Design review of the part built by this model. Coordinates are the model's own, in mm. Give positions to 0.01 mm unless a question says otherwise; leave off trailing zeros. Loops run counter-clockwise (first coordinate to the right, second up) from the corner with the lowest first, then second, coordinate; pieces in that order, holes last.
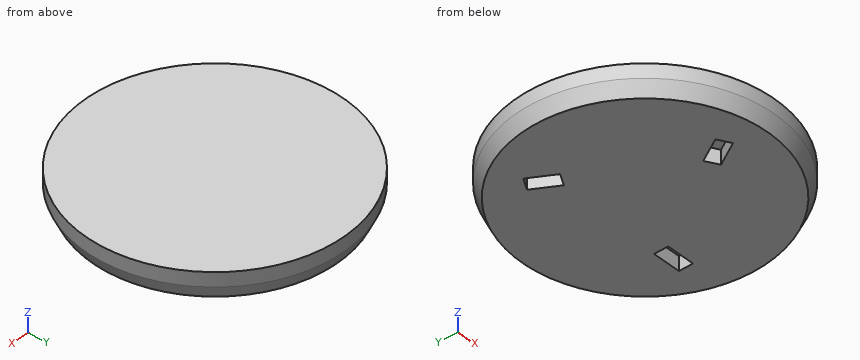
from build123d import *

# Parameters (mm, degrees)
F0_R     = 165
F1_DEPTH = 36
F2_W     = 36
F2_H     = 18
F3_DEPTH = 18
F4_SIZE2 = 8.393538
F4_SIZE  = 18


with BuildPart() as f1:
    # F0 (on Top) → F1 (new body)
    with BuildSketch(Plane.XY):
        Circle(F0_R)
    extrude(amount=F1_DEPTH)

    # F2 (on face) → F3 (cut)
    with BuildSketch(Plane(origin=(0, 0, 0), x_dir=(1, 0, 0), z_dir=(0, 0, -1))):
        Polygon((-9, 120.176915), (-24.588457, 111.176915), (-6.588457, 80), (9, 89), align=None)
        with Locations((90.576261, -43.294229)):
            Rectangle(F2_W, F2_H)
        Polygon((-81.576261, -36.705771), (-99.576261, -67.882686), (-83.987804, -76.882686), (-65.987804, -45.705771), align=None)
    extrude(amount=-F3_DEPTH, mode=Mode.SUBTRACT)

    # F4
    f4_edges = [f1.edges().sort_by_distance(p)[0] for p in [
        (-165, 0, 0),
    ]]
    chamfer(f4_edges, length=F4_SIZE, length2=F4_SIZE2)


solid = f1.part
Q1. Take a section at A-A (z = 12). Give the boundary of the cut face in (x, y).
Results:
outline: circle Ø324.4 at (0, 0); hole (-99.58, 67.88) - (-81.58, 36.71) - (-65.99, 45.71) - (-83.99, 76.88) - close; hole (-24.59, -111.18) - (-9, -120.18) - (9, -89) - (-6.59, -80) - close; hole (72.58, 34.29) - (108.58, 34.29) - (108.58, 52.29) - (72.58, 52.29) - close
Q2. Take a section at B-B (x = 0). Give the boundary of the cut face in (y, z).
Results:
outline: (-165, 18) - (-156.61, 0) - (-104.59, 0) - (-104.59, 18) - (-83.8, 18) - (-83.8, 0) - (156.61, 0) - (165, 18) - (165, 36) - (-165, 36) - close
Q3. Wall thickness on line 1 (Y direction, x = 76.5, z = 5); line 2 (Y direction, x = -96, z = 16); line 3 (X direction, y = -88, z = 12): over which ranges is each line inside the solid? List them lowest first.
Results:
line 1: y = -139.32 to 34.29, 52.29 to 139.32
line 2: y = -133.05 to 61.69, 69.95 to 133.05
line 3: x = -136.26 to -11.21, 7.27 to 136.26
Q4. Insertion check: pin 1 (10 mm diameter, centred on y = -127, z = 4.5, fed in from -X); pin 2 (3 mm diameter, centred on y = 129.5, z = 7.5, fed in from +X); pin 3 (9 mm diameter, centred on y = 40, z = 12.5, fed in from -X). Each pin has a flat end and moves straight along its axis. Give the tip position at first contact, or say it passes through.
Results:
pin 1: stops at x = -102.52
pin 2: stops at x = 96.49
pin 3: stops at x = -159.86
